For this review, take the finished solid that the model builds, in its own axes (mm). A direction names the side the tool comes from. Give positions to 0.01 mm unless a question says otherwise; leave off trailing zeros. Loops run counter-clockwise (first coordinate to the right, second up) from the corner with the lowest first, then second, coordinate; pieces in that order, holes last. Notation, with made-up numbers: (17, 76.25) -> (36, 76.25) arc R22 ccw to (36, 100.25) -> close; hole circle Ø10 at (-10, 89.5). An arc over 180 degrees is marked (long way). One line per question, with ' | ' between items. Start each with the question number.
(1) Draft analysis for pull direction Y (two halves, no side actions). For faces 3 (the cylindrical face through (0.385, -47.496, 1.479)), 4 (the flat face through (-17.5, 0, 1)), 5 (the cylindrical face through (-0.716, 35.453, 1.479)), state which applies: +Y half, -Y half, draft (parallel to the pull), parting line (faces both ways), or undercut.
(2) Tool access review of faces 1 (the flat face through (4, 9, 2)), 2 (the flat face through (17.5, 0, 1)): name each direction out of +Z, -Z, +X, -X, +Y, -Y from which nothing blocks a thin tool from reaching the whole face with its end or side.
(3) Consider section A-A (x = 0). Write out the cut boundary in (y, z).
(4) Consider section D-D (x = 14). Write out the cut boundary in (y, z), and give its area (3 significant figures).
(5) Wall thickness on probe 1 along Y at (x, z) = (0, 1.75); probe 2 along X at (y, z) = (10, 2.45); probe 3 along Y at (x, z) = (-1.5, 2.6): over which ranges is each line inside the solid? List them lowest first.
(6) Insertion check: P1, Ø1.5, axis at x = 2, z = 1, coming from the +Y side. The pin has a flat end and moves straight along its axis. Give the tip position at first contact, or say it passes through.
(7) Consider section B-B (z = 2.4). Write out the cut boundary in (x, y), and give its area (3 significant figures).
(8) Consider section C-C (y = 25.5). Write out the cut boundary in (x, z).
from build123d import *

# Parameters (mm, degrees)
CROQUIS1_R              = 5.5
CROQUIS1_R_2            = 3
SALIENTE_EXTRUIR1_DEPTH = 3
CORTAR_EXTRUIR1_REACH   = 52.71
CROQUIS2_W              = 8
CROQUIS2_H              = 3


with BuildPart() as part:
    # Croquis1 → Saliente-Extruir1 (new body)
    with BuildSketch(Plane.XY):
        with BuildLine():
            Line((-17.5, -30), (-17.5, 30))
            ThreePointArc((-17.5, 30), (0, 47.5), (17.5, 30))
            Line((17.5, 30), (17.5, -30))
            ThreePointArc((17.5, -30), (0, -47.5), (-17.5, -30))
        make_face()
        with Locations((0, 30)):
            Circle(CROQUIS1_R, mode=Mode.SUBTRACT)
        with Locations((0, -30)):
            Circle(CROQUIS1_R_2, mode=Mode.SUBTRACT)
    extrude(amount=SALIENTE_EXTRUIR1_DEPTH)

    # Croquis2 → Cortar-Extruir1 (cut, up to next)
    with BuildSketch(Plane.XY.offset(3), mode=Mode.PRIVATE) as cortar_extruir1_sk1:
        with Locations((0, 9.27)):
            Rectangle(CROQUIS2_W, CROQUIS2_H)
    cortar_extruir1_tool1 = extrude(cortar_extruir1_sk1.sketch, amount=-CORTAR_EXTRUIR1_REACH, mode=Mode.PRIVATE) & part.part
    add(cortar_extruir1_tool1.solids().sort_by_distance((0, 9.27, 3))[0], mode=Mode.SUBTRACT)


solid = part.part
A:
1) face 3: -Y half | face 4: draft | face 5: undercut
2) face 1: +Z, -Z | face 2: +Z, -Z, +X, +Y, -Y
3) outline: (-47.5, 0) -> (-33, 0) -> (-33, 3) -> (-47.5, 3) -> close; (-27, 0) -> (7.77, 0) -> (7.77, 3) -> (-27, 3) -> close; (10.77, 0) -> (24.5, 0) -> (24.5, 3) -> (10.77, 3) -> close; (35.5, 0) -> (47.5, 0) -> (47.5, 3) -> (35.5, 3) -> close
4) outline: (-40.5, 0) -> (40.5, 0) -> (40.5, 3) -> (-40.5, 3) -> close | area: 243 mm^2
5) probe 1: y = -47.5 to -33, -27 to 7.77, 10.77 to 24.5, 35.5 to 47.5 | probe 2: x = -17.5 to -4, 4 to 17.5 | probe 3: y = -47.44 to -32.6, -27.4 to 7.77, 10.77 to 24.71, 35.29 to 47.44
6) P1: stops at y = 47.46
7) outline: (-17.5, -30) arc R17.5 ccw to (17.5, -30) -> (17.5, 30) arc R17.5 ccw to (-17.5, 30) -> close; hole circle Ø11 at (0, 30); hole (-4, 7.77) -> (4, 7.77) -> (4, 10.77) -> (-4, 10.77) -> close; hole circle Ø6 at (0, -30) | area: 2,910 mm^2
8) outline: (-17.5, 0) -> (-3.16, 0) -> (-3.16, 3) -> (-17.5, 3) -> close; (3.16, 0) -> (17.5, 0) -> (17.5, 3) -> (3.16, 3) -> close
